```python
from build123d import *

# Parameters (mm, degrees)
SKETCH2_R           = 8.255
BOSS_EXTRUDE1_DEPTH = 6.35
SKETCH3_R           = 3.175
BOSS_EXTRUDE2_DEPTH = 3.81
SKETCH5_R           = 13.0175
SKETCH5_R_2         = 7.3025
BOSS_EXTRUDE5_DEPTH = 3.81
SKETCH4_R           = 13.6525
CUT_EXTRUDE1_DEPTH  = 3.81
SKETCH6_R           = 3.175
BOSS_EXTRUDE6_DEPTH = 3.81
SKETCH7_R           = 19.05
CUT_EXTRUDE2_DEPTH  = 31.75


with BuildPart() as part:
    # Sketch1 → Revolve1 (revolve)
    with BuildSketch(Plane.XY, mode=Mode.PRIVATE) as revolve1_sk:
        Polygon((0, 0), (59.69, 0), (59.69, 44.45), (53.34, 44.45), (53.34, 78.232), (21.59, 78.232), (21.59, 101.6), (2.54, 101.6), (2.54, 107.95), (76.2, 107.95), (76.2, 114.3), (82.55, 114.3), (82.55, 118.11), (72.39, 118.11), (72.39, 110.49), (-88.9, 110.49), (-88.9, 105.41), (-63.5, 105.41), (-63.5, 101.6), (-38.1, 101.6), (-38.1, 78.74), (-44.45, 78.74), (-44.45, 64.77), (-76.2, 64.77), (-76.2, 0), align=None)
    revolve(revolve1_sk.sketch.rotate(Axis((0, 0, 0), (1, 0, 0)), 90), axis=Axis((0, 0, 0), (1, 0, 0)))

    # Sketch2 → Boss-Extrude1 (add)
    with BuildSketch(Plane(origin=(21.59, 0, 0), x_dir=(0, 0, -1), z_dir=(1, 0, 0))):
        with Locations(Location((0, 88.9, 0), (0, 0, 180))):
            Circle(SKETCH2_R)
        with Locations(Location((44.45, 76.989658396, 0), (0, 0, 180))):
            Circle(SKETCH2_R)
        with Locations(Location((76.989658396, 44.45, 0), (0, 0, 180))):
            Circle(SKETCH2_R)
        with Locations(Location((88.9, 0, 0), (0, 0, 180))):
            Circle(SKETCH2_R)
        with Locations(Location((76.989658396, -44.45, 0), (0, 0, 180))):
            Circle(SKETCH2_R)
        with Locations(Location((44.45, -76.989658396, 0), (0, 0, 180))):
            Circle(SKETCH2_R)
        with Locations(Location((0, -88.9, 0), (0, 0, 180))):
            Circle(SKETCH2_R)
        with Locations(Location((-44.45, -76.989658396, 0), (0, 0, 180))):
            Circle(SKETCH2_R)
        with Locations(Location((-76.989658396, -44.45, 0), (0, 0, 180))):
            Circle(SKETCH2_R)
        with Locations(Location((-88.9, 0, 0), (0, 0, 180))):
            Circle(SKETCH2_R)
        with Locations(Location((-76.989658396, 44.45, 0), (0, 0, 180))):
            Circle(SKETCH2_R)
        with Locations(Location((-44.45, 76.989658396, 0), (0, 0, 180))):
            Circle(SKETCH2_R)
    extrude(amount=BOSS_EXTRUDE1_DEPTH)

    # Sketch3 → Boss-Extrude2 (add)
    with BuildSketch(Plane(origin=(53.34, 0, 0), x_dir=(0, 0, -1), z_dir=(1, 0, 0))):
        with Locations(Location((0, 60.325, 0), (0, 0, 180))):
            Circle(SKETCH3_R)
        with Locations(Location((30.1625, 52.242982483, 0), (0, 0, 180))):
            Circle(SKETCH3_R)
        with Locations(Location((52.242982483, 30.1625, 0), (0, 0, 180))):
            Circle(SKETCH3_R)
        with Locations(Location((60.325, 0, 0), (0, 0, 180))):
            Circle(SKETCH3_R)
        with Locations(Location((52.242982483, -30.1625, 0), (0, 0, 180))):
            Circle(SKETCH3_R)
        with Locations(Location((30.1625, -52.242982483, 0), (0, 0, 180))):
            Circle(SKETCH3_R)
        with Locations(Location((0, -60.325, 0), (0, 0, 180))):
            Circle(SKETCH3_R)
        with Locations(Location((-30.1625, -52.242982483, 0), (0, 0, 180))):
            Circle(SKETCH3_R)
        with Locations(Location((-52.242982483, -30.1625, 0), (0, 0, 180))):
            Circle(SKETCH3_R)
        with Locations(Location((-60.325, 0, 0), (0, 0, 180))):
            Circle(SKETCH3_R)
        with Locations(Location((-52.242982483, 30.1625, 0), (0, 0, 180))):
            Circle(SKETCH3_R)
        with Locations(Location((-30.1625, 52.242982483, 0), (0, 0, 180))):
            Circle(SKETCH3_R)
    extrude(amount=BOSS_EXTRUDE2_DEPTH)

    # Sketch5 → Boss-Extrude5 (add)
    # profile 1 of 3: a face of its own
    with BuildSketch(Plane(origin=(59.69, 0, 0), x_dir=(0, 0, -1), z_dir=(1, 0, 0))):
        with Locations(Location((0, 29.845, 0), (0, 0, 180))):
            Circle(SKETCH5_R)
        with Locations(Location((0, 29.845, 0), (0, 0, 180))):
            Circle(SKETCH5_R_2, mode=Mode.SUBTRACT)
    # profile 2 of 3: a face of its own
    with BuildSketch(Plane(origin=(59.69, 0, 0), x_dir=(0, 0, -1), z_dir=(1, 0, 0))):
        with Locations(Location((25.846528176, -14.9225, 0), (0, 0, 180))):
            Circle(SKETCH5_R)
        with Locations(Location((25.846528176, -14.9225, 0), (0, 0, 180))):
            Circle(SKETCH5_R_2, mode=Mode.SUBTRACT)
    # profile 3 of 3: a face of its own
    with BuildSketch(Plane(origin=(59.69, 0, 0), x_dir=(0, 0, -1), z_dir=(1, 0, 0))):
        with Locations(Location((-25.846528176, -14.9225, 0), (0, 0, 180))):
            Circle(SKETCH5_R)
        with Locations(Location((-25.846528176, -14.9225, 0), (0, 0, 180))):
            Circle(SKETCH5_R_2, mode=Mode.SUBTRACT)
    extrude(amount=BOSS_EXTRUDE5_DEPTH)

    # Sketch4 → Cut-Extrude1 (cut)
    with BuildSketch(Plane(origin=(59.69, 0, 0), x_dir=(0, 0, -1), z_dir=(1, 0, 0))):
        Circle(SKETCH4_R)
    extrude(amount=-CUT_EXTRUDE1_DEPTH, mode=Mode.SUBTRACT)

    # Sketch6 → Boss-Extrude6 (add)
    with BuildSketch(Plane.ZY.offset(44.45)):
        with Locations(Location((0, 69.85, 0), (0, 0, 180))):
            Circle(SKETCH6_R)
        with Locations(Location((34.925, 60.491874454, 0), (0, 0, 180))):
            Circle(SKETCH6_R)
        with Locations(Location((60.491874454, 34.925, 0), (0, 0, 180))):
            Circle(SKETCH6_R)
        with Locations(Location((69.85, 0, 0), (0, 0, 180))):
            Circle(SKETCH6_R)
        with Locations(Location((60.491874454, -34.925, 0), (0, 0, 180))):
            Circle(SKETCH6_R)
        with Locations(Location((34.925, -60.491874454, 0), (0, 0, 180))):
            Circle(SKETCH6_R)
        with Locations(Location((0, -69.85, 0), (0, 0, 180))):
            Circle(SKETCH6_R)
        with Locations(Location((-34.925, -60.491874454, 0), (0, 0, 180))):
            Circle(SKETCH6_R)
        with Locations(Location((-60.491874454, -34.925, 0), (0, 0, 180))):
            Circle(SKETCH6_R)
        with Locations(Location((-69.85, 0, 0), (0, 0, 180))):
            Circle(SKETCH6_R)
        with Locations(Location((-60.491874454, 34.925, 0), (0, 0, 180))):
            Circle(SKETCH6_R)
        with Locations(Location((-34.925, 60.491874454, 0), (0, 0, 180))):
            Circle(SKETCH6_R)
    extrude(amount=BOSS_EXTRUDE6_DEPTH)

    # Sketch7 → Cut-Extrude2 (cut)
    with BuildSketch(Plane.ZY.offset(76.2)):
        Circle(SKETCH7_R)
    extrude(amount=-CUT_EXTRUDE2_DEPTH, mode=Mode.SUBTRACT)


solid = part.part
```
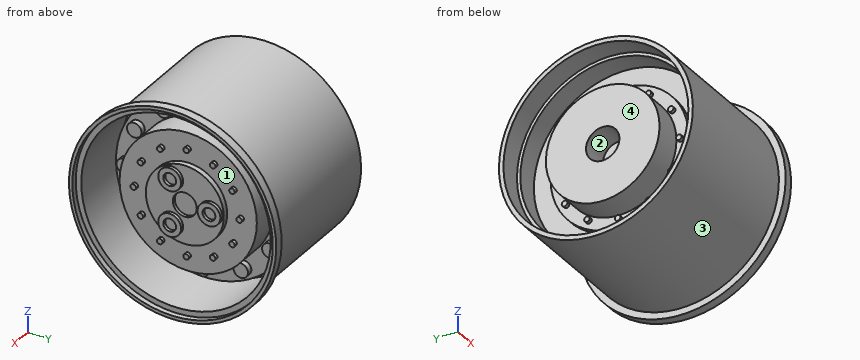
The model under review builds one solid part; all positions refer to its coordinate system, in mm. Face numbers are marked on the shaded views. A direction names the side the tool comes from. Round coordinates to 2 decimals unless told otherwise and drop trailing zeros. Order: outer loops, then holes, each group sorted by start corner. A loop starts at its lowest first (then second) coordinate and runs counter-clockwise, first axis right, second up. Notation, with made-up numbers: M 30,73.25 L 42,73.25 A30 cw 42,102.25 Z; hole C 28.25,-32 d4. An arc over 180 degrees is marked long. Use a Markdown table: item, result.
1) Tool access review of the marked faces 1 and 2: name each direction out of +Z, -Z, +X, -X, +Y, -Y from which nothing blocks a thin tool from reaching the whole face with its end or side.
Report:
| item | result |
|---|---|
| face 1 | +X |
| face 2 | -X |
2) Draft analysis for pull direction Z (two halves, no side actions). For the marked faces 3 and 4, state which applies: released by +Z, released by -Z, zero draft, split by the parting line, or undercut.
Report:
| item | result |
|---|---|
| face 3 | split by the parting line |
| face 4 | undercut |
3) Consider section D-D (x = 13.5). Write out the cut boundary in (y, z), then the cut area to 3 significant figures.
Report:
| item | result |
|---|---|
| outline | C 0,0 d220.98; C 0,0 d203.2; hole C 0,0 d215.9 |
| area | 34,200 mm^2 |
4) Consider section A-A (x = 31). Write out the cut boundary in (y, z), then the cut area to 3 significant figures.
Report:
| item | result |
|---|---|
| outline | C 0,0 d220.98; C 0,0 d156.46; hole C 0,0 d215.9 |
| area | 21,000 mm^2 |
5) Insertion check: pin 1 (10 mm diameter, centred on x = 45, y = -51, fed in from +Z); pin 2 (18 mm diameter, centred on y = -90, z = -1, fed in from +X); pin 3 (7 mm diameter, centred on y = 33.5, z = -61, fed in from -X). Each pin has a flat end and moves straight along its axis. Give the tip position at first contact, or say it passes through.
Report:
| item | result |
|---|---|
| pin 1 | z = 100.46 |
| pin 2 | x = 27.94 |
| pin 3 | x = -48.26 |
6) Wall thickness on line 1 along Y through (x, z) = (58, 0); line 2 along Y through (x, z) = (-51.5, 0); line 3 along Z through (x, y) = (12, 33): over which ranges is each line inside the solid? List them lowest first. Write a range as [from, to].
Report:
| item | result |
|---|---|
| line 1 | [-110.49, -107.95], [-44.45, -13.65], [13.65, 44.45], [107.95, 110.49] |
| line 2 | [-110.49, -101.6], [-64.77, -19.05], [19.05, 64.77], [101.6, 110.49] |
| line 3 | [-105.45, -102.78], [-96.09, 96.09], [102.78, 105.45] |
